Check sheet for the modelled part. Datum: model origin and axes. Units: mm. Face numbers are marked on the shaded views. A direction names the side the tool comes from. Round coordinates to 2 decimals unless told otherwise and drop trailing zeros. Order: outer loops, then holes, each group sorted by start corner. A loop starts at its lowest first (then second) coordinate and runs counter-clockwise, first axis right, second up. Notation, with made-up numbers: (-28, -32.5) -> (26, -32.5) arc R22 ccw to (26, -19.5) -> close; hole circle Ø3 at (34.5, 3.25). An arc over 180 degrees is marked (long way). Answer in a Markdown table with one row per item.
```python
from build123d import *

# Parameters (mm, degrees)
F0_R      = 11.6
F1_DEPTH  = 2
F3_DEPTH  = 5
F5_DEPTH  = 10
F6_W      = 0.8
F6_H      = 5
F7_DEPTH  = 5
F8_R      = 8.8
F9_DEPTH  = 6
F10_SIZE2 = 0.99999
F10_SIZE  = 2.79999
F11_R     = 2
F12_SIZE2 = 0.5
F12_SIZE  = 1.5
F13_R     = 0.9
F14_DEPTH = 22.4013731274


# Not quite as in the source:
# - a fillet or chamfer is up to 0.001 mm smaller than in the source, because OpenCascade refuses the exact size


with BuildPart() as f1:
    # F0 (on Top) → F1 (new body)
    with BuildSketch(Plane.XY):
        Circle(F0_R)
    extrude(amount=F1_DEPTH)

    # F2 (on face) → F3 (join)
    with BuildSketch(Plane(origin=(0, 0, 0), x_dir=(1, 0, 0), z_dir=(0, 0, -1))):
        with BuildLine():
            Line((-9.05, -2.5), (-9.05, -4.4841387133))
            ThreePointArc((-9.05, -4.4841387133), (0, -10.1), (9.05, -4.4841387133))
            Line((9.05, -4.4841387133), (9.05, -2.5))
            Line((9.05, -2.5), (9.05, 2.5))
            Line((9.05, 2.5), (9.05, 4.4841387133))
            ThreePointArc((9.05, 4.4841387133), (5.7442463725, 8.3074444694), (1, 10.0503731274))
            Line((1, 10.0503731274), (1, 10.8003731274))
            Line((1, 10.8003731274), (-1, 10.8003731274))
            Line((-1, 10.8003731274), (-1, 10.0503731274))
            ThreePointArc((-1, 10.0503731274), (-5.7442463725, 8.3074444694), (-9.05, 4.4841387133))
            Line((-9.05, 4.4841387133), (-9.05, 2.5))
            Line((-9.05, 2.5), (-9.05, -2.5))
        make_face()
        with BuildLine():
            Line((-9.7857038582, -2.5), (-9.05, -2.5))
            Line((-9.05, -2.5), (-9.05, 2.5))
            Line((-9.05, 2.5), (-9.7857038582, 2.5))
            ThreePointArc((-9.7857038582, 2.5), (-10.1, 0), (-9.7857038582, -2.5))
        make_face()
        with BuildLine():
            Line((9.05, 2.5), (9.05, -2.5))
            Line((9.05, -2.5), (9.7857038582, -2.5))
            ThreePointArc((9.7857038582, -2.5), (10.1, 0), (9.7857038582, 2.5))
            Line((9.7857038582, 2.5), (9.05, 2.5))
        make_face()
    extrude(amount=F3_DEPTH)

    # F4 (on face) → F5 (join)
    with BuildSketch(Plane(origin=(0, 0, -5), x_dir=(1, 0, 0), z_dir=(0, 0, -1))):
        with BuildLine():
            Line((6.5, 6.3), (-6.5, 6.3))
            ThreePointArc((-6.5, 6.3), (-7.9142135624, 5.7142135624), (-8.5, 4.3))
            Line((-8.5, 4.3), (-8.5, -4.3))
            ThreePointArc((-8.5, -4.3), (-7.9142135624, -5.7142135624), (-6.5, -6.3))
            Line((-6.5, -6.3), (6.5, -6.3))
            ThreePointArc((6.5, -6.3), (7.9142135624, -5.7142135624), (8.5, -4.3))
            Line((8.5, -4.3), (8.5, 4.3))
            ThreePointArc((8.5, 4.3), (7.9142135624, 5.7142135624), (6.5, 6.3))
        make_face()
    extrude(amount=F5_DEPTH)

    # F6 (on face) → F7 (cut)
    with BuildSketch(Plane(origin=(0, 0, -15), x_dir=(1, 0, 0), z_dir=(0, 0, -1))):
        Rectangle(F6_W, F6_H)
        with Locations((-7.35, 0)):
            Rectangle(F6_W, F6_H)
        with Locations((7.35, 0)):
            Rectangle(F6_W, F6_H)
    extrude(amount=-F7_DEPTH, mode=Mode.SUBTRACT)

    # F8 (on face) → F9 (cut)
    with BuildSketch(Plane.XY.offset(2)):
        Circle(F8_R)
    extrude(amount=-F9_DEPTH, mode=Mode.SUBTRACT)

    # F10 (size 2.8 and 1 in the source; OpenCascade refuses exactly that, so slightly less here)
    f10_edges = [f1.edges().sort_by_distance(p)[0] for p in [
        (-11.6, 0, 2),
    ]]
    f10_side = f1.faces().sort_by_distance((-11.271902, 0, 2))[0]
    chamfer(f10_edges, length=F10_SIZE, length2=F10_SIZE2, reference=f10_side)

    # F11
    f11_edges = [f1.edges().sort_by_distance(p)[0] for p in [
        (-9.05, 4.484139, -2.5),
        (-9.05, -4.484139, -2.5),
        (9.05, -4.484139, -2.5),
        (9.05, 4.484139, -2.5),
    ]]
    fillet(f11_edges, radius=F11_R)

    # F12
    f12_edges = [f1.edges().sort_by_distance(p)[0] for p in [
        (0, -10.800373, -5),
    ]]
    f12_side = f1.faces().sort_by_distance((0, -10.800373, -2.5))[0]
    chamfer(f12_edges, length=F12_SIZE, length2=F12_SIZE2, reference=f12_side)

    # F13 (on face) → F14 (cut, through all)
    with BuildSketch(Plane.XZ.offset(10.8003731274)):
        with Locations((0, -1.4)):
            Circle(F13_R)
    extrude(amount=-F14_DEPTH, mode=Mode.SUBTRACT)


solid = f1.part
```
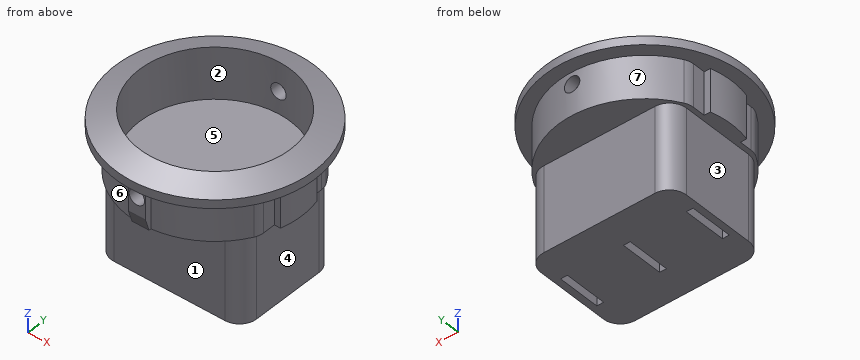
(1) Draft check along Y on the marked faces 1, 2 and 3. Enter one of: pulls with the +Y half, pulls with the -Y half, needs draft (parallel to the pull), parting line crosses it, or undercut.
Solutions:
| item | result |
|---|---|
| face 1 | pulls with the -Y half |
| face 2 | undercut |
| face 3 | needs draft |
(2) Depth check by flat-ended pin: pin 1 Ø8 at (x, y) = (3.5, -7) entering from +Z; pin 2 Ø3 at (x, z) = (-4, -2.5) entering from +Y; pin 3 Ø0.7 at (y, z) = (-3, -3) entering from +X; pin 4 Ø1.5 at (x, z) = (8, -13) entering from -Y. Enter the tip coordinate at first touch or a pass-through.
Solutions:
| item | result |
|---|---|
| pin 1 | z = 2 |
| pin 2 | y = 9.79 |
| pin 3 | x = 9.05 |
| pin 4 | y = -6.15 |
(3) Section check D-D on z = -5.5. Record the boundary of the cut face in (x, y), plus the area to 3 significant figures.
Solutions:
| item | result |
|---|---|
| outline | (-8.5, -4.3) arc R2 ccw to (-6.5, -6.3) -> (6.5, -6.3) arc R2 ccw to (8.5, -4.3) -> (8.5, 4.3) arc R2 ccw to (6.5, 6.3) -> (-6.5, 6.3) arc R2 ccw to (-8.5, 4.3) -> close |
| area | 211 mm^2 |
(4) Scan lines: probe 1 along X at (y, z) = (0.25, -8.5); probe 2 along Z at (x, y) = (-4.25, -4); probe 3 along Z at (x, y) = (0, 9.25). Record each from-to range of solid material in increasing order. Write a range as from..to.
Solutions:
| item | result |
|---|---|
| probe 1 | -8.5..8.5 |
| probe 2 | -15..-4 |
| probe 3 | -5..-2.3, -0.5..1.84 |
(5) Section check C-C on z = -12.5. Record the boundary of the cut face in (x, y), plus the area to 3 significant figures.
Solutions:
| item | result |
|---|---|
| outline | (-8.5, -4.3) arc R2 ccw to (-6.5, -6.3) -> (6.5, -6.3) arc R2 ccw to (8.5, -4.3) -> (8.5, 4.3) arc R2 ccw to (6.5, 6.3) -> (-6.5, 6.3) arc R2 ccw to (-8.5, 4.3) -> close; hole (-7.75, -2.5) -> (-6.95, -2.5) -> (-6.95, 2.5) -> (-7.75, 2.5) -> close; hole (-0.4, -2.5) -> (0.4, -2.5) -> (0.4, 2.5) -> (-0.4, 2.5) -> close; hole (6.95, -2.5) -> (7.75, -2.5) -> (7.75, 2.5) -> (6.95, 2.5) -> close |
| area | 199 mm^2 |
(6) Tool access check on the marked faces 4, 5, 6 and 7. Record the directions out of +Z, -Z, +X, -X, +Y, -Y that give a thin tool (end or side, any length) a straight path to the whole face; none if there is none.
Solutions:
| item | result |
|---|---|
| face 4 | -Z, +X, +Y, -Y |
| face 5 | +Z |
| face 6 | -Z, -X, -Y |
| face 7 | -Z, +Y |
(7) Section check A-A on x = 0. Give the number of separate pieces and of enclosed holes in the cut face, plus the area to 3 significant figures.
Solutions:
| item | result |
|---|---|
| separate pieces | 3 |
| enclosed holes | 0 |
| area | 137 mm^2 |
